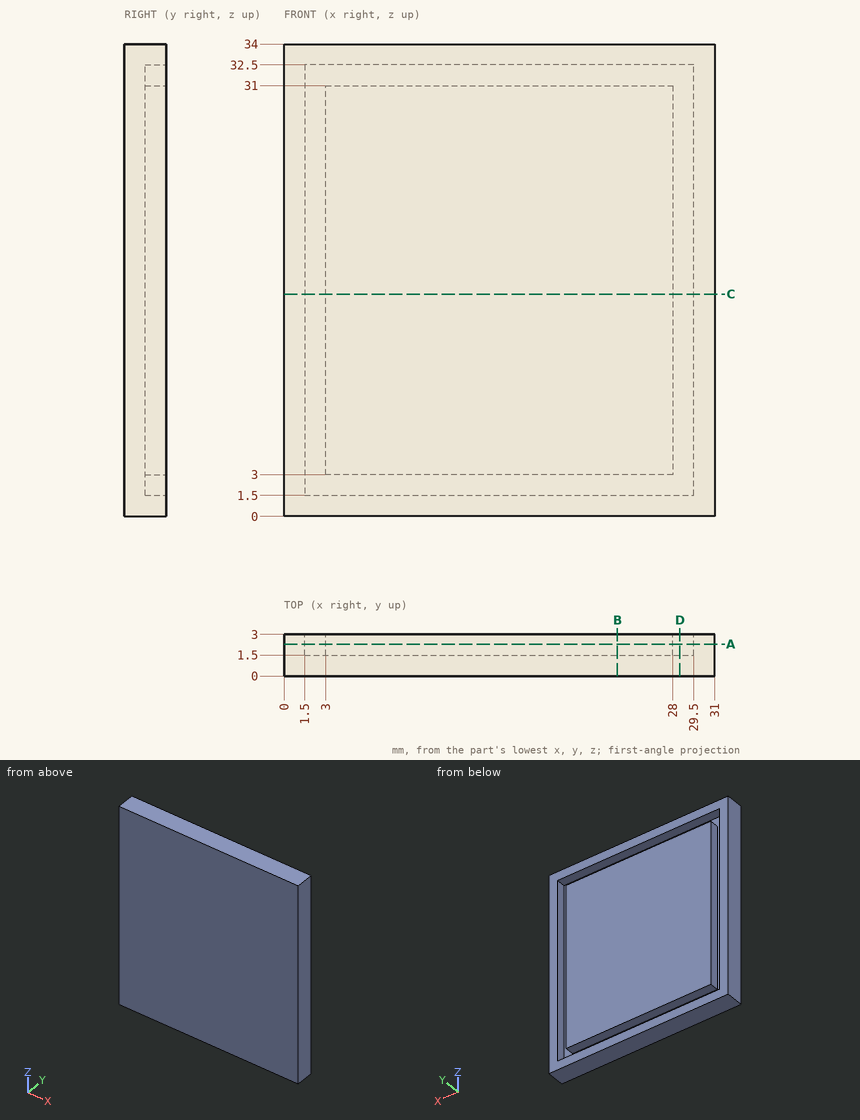
The figure shows three views and two pictorial views of one solid part (mm, origin at its lowest corner). Answer the questions. Coordinates: 2 decimals unless noted, no trailing zeros. Write each loop counter-clockwise with the first axis right and the second up, starting at its lowest first coordinate (ties: lowest second). Pieces come first, ordered by that corner, then holes. Notation, with made-up numbers: M 0,-25.5 L 49,-25.5 A22 ccw 49,13.5 Z; hole C 69.5,-2.5 d8. An arc over 180 degrees is marked long. Answer as CSV lines item,"result". Start each with the question number.
Item 1: Consider L1, parallel to Z at x = 10.5, y = 2.1; L2, parallel to X at y = 2.45, z = 19.5; L3, parallel to Z at x = 2, y = 2. Determine where each line is inside the solid, lowest interval first.
Item 2: Section D-D on x = 28.5 is taken. Write down the section's boundary in (y, z).
Item 3: Section C-C on z = 16 is taken. Write down the section's boundary in (x, y), and give its area (3 significant figures).
Item 4: Section B-B on x = 24 is taken. Write down the section's boundary in (y, z).
Item 5: Section A-A on y = 2.3 is taken. Write down the section's boundary in (x, z).
Checks:
1,L1,"z = 0 to 1.5, 3 to 31, 32.5 to 34"
1,L2,"x = 0 to 1.5, 3 to 28, 29.5 to 31"
1,L3,"z = 0 to 1.5, 32.5 to 34"
2,outline,"M 0,0 L 3,0 L 3,1.5 L 1.5,1.5 L 1.5,32.5 L 3,32.5 L 3,34 L 0,34 Z"
3,outline,"M 0,0 L 31,0 L 31,3 L 29.5,3 L 29.5,1.5 L 28,1.5 L 28,3 L 3,3 L 3,1.5 L 1.5,1.5 L 1.5,3 L 0,3 Z"
3,area,"88.5 mm²"
4,outline,"M 0,0 L 3,0 L 3,1.5 L 1.5,1.5 L 1.5,3 L 3,3 L 3,31 L 1.5,31 L 1.5,32.5 L 3,32.5 L 3,34 L 0,34 Z"
5,outline,"M 0,0 L 31,0 L 31,34 L 0,34 Z; M 3,3 L 28,3 L 28,31 L 3,31 Z; hole M 1.5,1.5 L 29.5,1.5 L 29.5,32.5 L 1.5,32.5 Z"
